Here's how the part is built. I have some questions about the finished solid (model axes, mm). A direction names the side the tool comes from. Give positions to 0.01 mm unless a question says otherwise; leave off trailing zeros. Write each loop counter-clockwise with the first axis right and the second up, starting at its lowest first coordinate (ties: lowest second). Pieces come first, ordered by that corner, then holes. Notation, with made-up numbers: (88.5, 56) -> (138.5, 56) arc R5 ccw to (138.5, 61) -> close; hole circle Ø8 at (49.5, 56). An arc over 180 degrees is marked (long way). Use one line per item in the form item = value.
```python
from build123d import *

# Parameters (mm, degrees)
FILETE1_R      = 1
FILETE2_R      = 1
CHANFRO1_SIZE  = 1.5
CHANFRO1_SIZE2 = 0.866025404


with BuildPart() as part:
    # Esboço1 → Revolução1 (revolve)
    with BuildSketch(Plane.XY, mode=Mode.PRIVATE) as revolu_o1_sk:
        Polygon((0, 44.337029737), (7.5, 44.337029737), (9.5, 43.837029737), (9.5, 40.337029737), (7, 40.337029737), (7, 32.337029737), (6.5, 32.337029737), (6.5, 26.337029737), (6, 24.337029737), (6, -4.662970263), (0, -4.662970263), align=None)
    revolve(revolu_o1_sk.sketch.rotate(Axis((0, -66.826190476, 0), (0, 1, 0)), 90), axis=Axis((0, -66.826190476, 0), (0, 1, 0)))

    # Filete1
    filete1_edges = [part.edges().sort_by_distance(p)[0] for p in [
        (0, 43.837029737, 9.5),
    ]]
    fillet(filete1_edges, radius=FILETE1_R)

    # Filete2
    filete2_edges = [part.edges().sort_by_distance(p)[0] for p in [
        (0, 40.337029737, 9.5),
    ]]
    fillet(filete2_edges, radius=FILETE2_R)

    # Chanfro1
    chanfro1_edges = [part.edges().sort_by_distance(p)[0] for p in [
        (0, -4.662970263, 6),
    ]]
    chanfro1_side = [part.faces().sort_by_distance(p)[0] for p in [
        (0, 9.837029737, 6),
    ]]
    chamfer(chanfro1_edges, length=CHANFRO1_SIZE, length2=CHANFRO1_SIZE2, reference=chanfro1_side[0])


solid = part.part
```
Q1. If I drill on line 1 along Y through (x, z) = (-3.5, -7); line 2 along Y through (x, z) = (4, -7.75); line 3 along X through (y, z) = (11, -3), over which ranges is the centre line in solid material (lowest first)? Write a range as from..to.
Result set:
line_1 = 40.34..44.26
line_2 = 40.36..44.03
line_3 = -5.2..5.2
Q2. Which directions (+Z, -Z, +X, -X, +Y, -Y) give clear straight access to the entire face, cutting with the end or side of a thin tool? Please do faces 1 (the face through (6.21, 36.28, -3.23)), 2 (the face through (0, -4.663, 0)).
Result set:
face_1 = -Y
face_2 = +Z, -Z, +X, -X, -Y
Q3. Will these pins go through, and if not, where does the flat tip stop? pin 1 Ø1 at (x, y) = (-1.5, 31) entering from +Z; pin 2 Ø4 at (y, z) = (12, 3) entering from -X; pin 3 Ø6 at (x, y) = (-1, 7) entering from -Z.
Result set:
pin_1 = 6.42
pin_2 = -5.92
pin_3 = -6
Q4. I want a section at B-B, the plane y = 37. Write out the boundary of the cut face in (x, z).
Result set:
outline = circle Ø14 at (0, 0)
Q5. I want a section at A-A, the plane y = 8.5. Write out the boundary of the cut face in (x, z), and give its area (3 significant figures).
Result set:
outline = circle Ø12 at (0, 0)
area = 113 mm2
